```python
from build123d import *

# Parameters (mm, degrees)
BOSS_EXTRUDE1_DEPTH       = 180.975
SKETCH3_W                 = 3.175
SKETCH3_H                 = 3.175
CUT_EXTRUDE2_DEPTH        = 185.505475867
F_8_32_TAPPED_HOLE1_D     = 3.4544
F_8_32_TAPPED_HOLE2_D     = 3.4544
F_8_32_TAPPED_HOLE2_DEPTH = 10.668
F_8_32_TAPPED_HOLE2_TIP   = 1.037806461
FILLET1_R                 = 3.175
FILLET2_R                 = 2.3622


with BuildPart() as part:
    # Sketch1 → Boss-Extrude1 (new, symmetric)
    with BuildSketch(Plane(origin=(0, 0, 0), x_dir=(0, 0, -1), z_dir=(1, 0, 0))):
        Polygon((0, 0), (0, 25.4), (3.175, 25.4), (3.175, 3.175), (25.4, 3.175), (25.4, 0), align=None)
    extrude(amount=BOSS_EXTRUDE1_DEPTH, both=True)

    # Sketch3 → Cut-Extrude2 (cut, through all)
    with BuildSketch(Plane(origin=(0, 0, -25.4), x_dir=(-1, 0, 0), z_dir=(0, 0, -1))):
        with Locations((-179.3875, 1.5875)):
            Rectangle(SKETCH3_W, SKETCH3_H)
    cut_extrude2 = extrude(amount=-CUT_EXTRUDE2_DEPTH, mode=Mode.SUBTRACT)

    # Mirror2: Cut-Extrude2 across plane
    add(cut_extrude2.mirror(Plane(origin=(0, 0, 0), x_dir=(0, 0, 1), z_dir=(1, 0, 0))), mode=Mode.SUBTRACT)

    # #8-32 Tapped Hole1 (through all)
    with Locations(Plane.XY):
        with Locations((109.4105, 15.875), (45.9105, 15.875), (-17.5895, 15.875)):
            Hole(F_8_32_TAPPED_HOLE1_D / 2)

    # #8-32 Tapped Hole2
    with Locations(Plane(origin=(0, 3.175, 0), x_dir=(-1, 0, 0), z_dir=(0, 1, 0))):
        with Locations((131.953, -13.335), (-131.953, -13.335)):
            Hole(F_8_32_TAPPED_HOLE2_D / 2, depth=F_8_32_TAPPED_HOLE2_DEPTH)
            with Locations((0, 0, -(F_8_32_TAPPED_HOLE2_DEPTH + F_8_32_TAPPED_HOLE2_TIP / 2))):  # 118° drill point
                Cone(0, F_8_32_TAPPED_HOLE2_D / 2, F_8_32_TAPPED_HOLE2_TIP, mode=Mode.SUBTRACT)

    # Fillet1
    fillet1_edges = [part.edges().sort_by_distance(p)[0] for p in [
        (0, 3.175, -3.175),
    ]]
    fillet(fillet1_edges, radius=FILLET1_R)

    # Fillet2
    fillet2_edges = [part.edges().sort_by_distance(p)[0] for p in [
        (0, 25.4, -3.175),
        (0, 3.175, -25.4),
    ]]
    fillet(fillet2_edges, radius=FILLET2_R)


solid = part.part
```
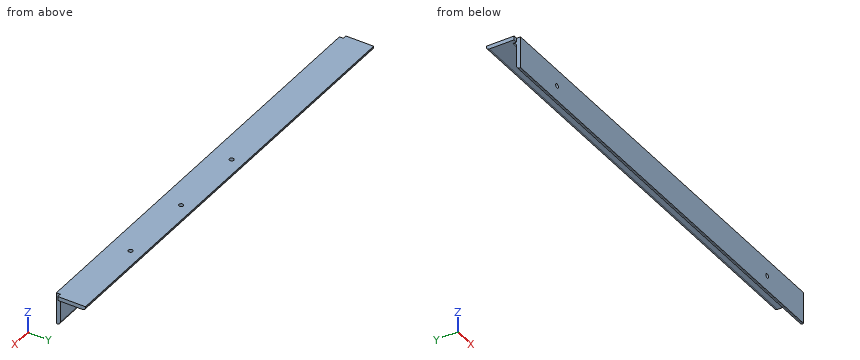
Source: CAD feature listing. Evaluate the final solid. Frame: model axes, mm. Coordinates: 2 decimals unless noted, no trailing zeros. Loops run counter-clockwise (first coordinate to the right, second up) from the corner with the lowest first, then second, coordinate; pieces in that order, holes last. Notation, with made-up numbers: M 40.5,33.25 L 81.5,33.25 A30 ccw 81.5,58.25 Z; hole C 37.5,31.5 d1. An arc over 180 degrees is marked long. Use a Markdown table: item, result. Add a question column.
Q1. Material intervals for L1, parallel to Z at x = -9.5, y = 20.5 (3 decimals); L2, parallel to Y at x = -134, z = -8.75 (3 decimals); L3, parallel to X at y = 2, z = -19.25, sorted ascending.
Q2. Section query A-A, the plane x = 27.5. Return loops of the section in (y, z) (3 decimals).
Q3. First-contact query: pin 1 (6 mm diameter, centred on x = 135, z = -8.5, fed in from +Y); pin 2 (4 mm diameter, centred on x = 131.953, z = -13.335, fed in from +Y) (3 decimals); pin 3 (3 mm diameter, centred on y = 4.5, z = -7, fed in from -X). Flat tips, straight axial feed; report the tip coordinate or a pass-through.
Result:
| question | item | result |
|---|---|---|
| 1 | L1 | z = -3.175 to 0 |
| 1 | L2 | y = 0 to 3.175 |
| 1 | L3 | x = -177.8 to 177.8 |
| 2 | outline | M 0,-25.4 L 0.813,-25.4 A2.362 ccw 3.175,-23.038 L 3.175,-6.35 A3.175 cw 6.35,-3.175 L 23.038,-3.175 A2.362 ccw 25.4,-0.813 L 25.4,0 L 0,0 Z |
| 3 | pin 1 | stops at y = 3.29 |
| 3 | pin 2 | stops at y = 3.175 |
| 3 | pin 3 | stops at x = -177.8 |
